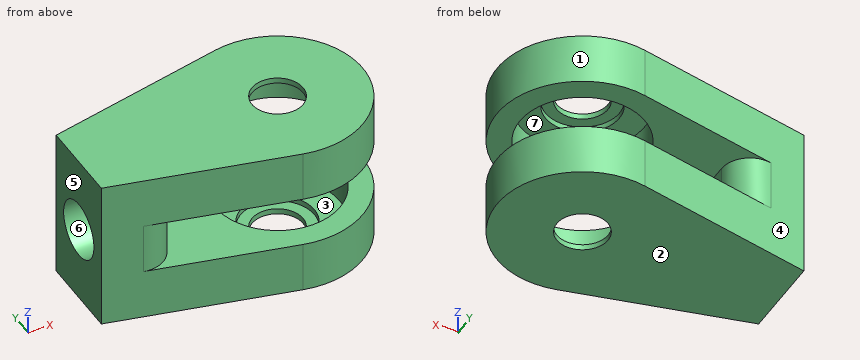
from build123d import *

# Parameters (mm, degrees)
SKETCH1_R               = 15
BOSS_EXTRUDE1_DEPTH     = 9
SKETCH2_R               = 11
CUT_EXTRUDE1_DEPTH      = 7
CUT_EXTRUDE2_REACH      = 40.717
SKETCH3_R               = 4.5
BOSS_EXTRUDE3_REACH     = 44.119
SKETCH6_R               = 5.031250000000002
CUT_EXTRUDE3_DEPTH      = 11.43
FILLET1_R               = 5
CUT_EXTRUDE4_DEPTH      = 1
CUT_EXTRUDE4_DEPTH_BACK = 24
SKETCH7_R               = 6.5


with BuildPart() as part:
    # Sketch1 → Boss-Extrude1 (new body)
    with BuildSketch(Plane.XY):
        with BuildLine():
            ThreePointArc((-3.2926829268292646, -14.634146341463415), (-15, 1.84e-15), (-3.2926829268292708, 14.634146341463413))
            Line((-3.2926829268292703, 14.634146341463419), (-35.00000000000001, 7.499999999999995))
            Line((-35.00000000000001, 7.499999999999995), (-35, -7.500000000000005))
            Line((-35, -7.500000000000005), (-3.292682926829265, -14.634146341463415))
        make_face()
        Circle(SKETCH1_R)
    extrude(amount=BOSS_EXTRUDE1_DEPTH)

    # Sketch2 → Cut-Extrude1 (cut)
    with BuildSketch(Plane.XY.offset(9)):
        Circle(SKETCH2_R)
    extrude(amount=-CUT_EXTRUDE1_DEPTH, mode=Mode.SUBTRACT)

    # Sketch3 → Cut-Extrude2 (cut, up to next)
    with BuildSketch(Plane.XY.offset(2), mode=Mode.PRIVATE) as cut_extrude2_sk1:
        Circle(SKETCH3_R)
    cut_extrude2_tool1 = extrude(cut_extrude2_sk1.sketch, amount=-CUT_EXTRUDE2_REACH, mode=Mode.PRIVATE) & part.part
    add(cut_extrude2_tool1.solids().sort_by_distance((0, 0, 2))[0], mode=Mode.SUBTRACT)


with BuildPart() as body_2:
    # Mirror8: mirrored copy
    add(part.part.mirror(Plane.XY.offset(13.499999999999998)))

    # Sketch4 → Boss-Extrude3 (add, up to next)
    with BuildSketch(Plane.XY.offset(9), mode=Mode.PRIVATE) as boss_extrude3_sk1:
        Polygon((-35.00000000000001, 7.499999999999995), (-35.00000000000001, -7.500000000000005), (-22.300000000000008, -10.357500000000002), (-22.300000000000015, 10.357499999999998), align=None)
    boss_extrude3_tool1 = extrude(boss_extrude3_sk1.sketch, amount=BOSS_EXTRUDE3_REACH, mode=Mode.PRIVATE) - body_2.part

    add(part.part)  # Boss-Extrude3 merges part
    add(boss_extrude3_tool1.solids().sort_by_distance((-28.311298, 0, 9))[0])

    # Sketch6 → Cut-Extrude3 (cut)
    with BuildSketch(Plane.ZY.offset(35.00000000000001)):
        with Locations((13.499999999999998, -3.47e-15)):
            Circle(SKETCH6_R)
    extrude(amount=-CUT_EXTRUDE3_DEPTH, mode=Mode.SUBTRACT)

    # Fillet1
    fillet1_edges = [body_2.edges().sort_by_distance(p)[0] for p in [
        (-22.300000000000015, 10.357499999999996, 13.499999999999998),
        (-22.300000000000008, -10.3575, 13.499999999999998),
    ]]
    fillet(fillet1_edges, radius=FILLET1_R)

    # Sketch7 → Cut-Extrude4 (cut, two sides: drawn at the far end of the back side and taken through both)
    with BuildSketch(Plane.XY.offset(24.999999999999993).offset(-CUT_EXTRUDE4_DEPTH_BACK)):
        Circle(SKETCH7_R)
    extrude(amount=CUT_EXTRUDE4_DEPTH + CUT_EXTRUDE4_DEPTH_BACK, mode=Mode.SUBTRACT)


solid = body_2.part
Design review of the part built by this model. Coordinates are the model's own, in mm. Face numbers are marked on the shaded views. A direction names the side the tool comes from. Round coordinates to 2 decimals unless told otherwise and drop trailing zeros. Order: outer loops, then holes, each group sorted by start corner. A loop starts at its lowest first (then second) coordinate and runs counter-clockwise, first axis right, second up. Notation, with made-up numbers: M -26,72.5 L -5,72.5 A19 ccw -5,80.5 Z; hole C 45,23 d4. An arc over 180 degrees is marked long. Answer as CSV lines item,"result". Start each with the question number.
1) Add section A-A (x = 0). Give the number of separate pieces and of enclosed holes in the cut face, then the cut area to 3 significant figures.
2) Add section C-C (z = 20.75). Give the boundary of the cut face in (x, y), then the cut area to 3 significant figures.
3) Add section B-B (y = 12). Give the boundary of the cut face in (x, z).
4) Wall thickness on line 1 along Z through (x, y) = (-4, -3.5); line 2 along X through (y, z) = (0, 26.65); line 3 along Z through (x, y) = (-21.5, -10.5): over which ranges is each line inside the solid? List them lowest first. Write a range as [from, to].
5) For pin 1 Ø8 at (y, z) = (-2.5, 18.5) entering from +X; pin 2 Ø5 at (y, z) = (-10.5, 8.5) entering from +X; pin 3 Ø6 at (y, z) = (0, 13.5) entering from -X; pin 4 Ø6 at (y, z) = (8.5, 18.5) entering from +X, all flat-tipped, find the tip position at first contact; note any pin that passes through.
6) The part is to be moulded in two halves that separate along Y. For the marked faces 1, 2, 3 and 4, say which applies: +Y half, -Y half, draft (parallel to the pull), parting line (faces both ways), or undercut.
7) Tool access review of the marked faces 5, 6 and 7: name each direction out of +Z, -Z, +X, -X, +Y, -Y from which nothing blocks a thin tool from reaching the whole face with its end or side.
8) Add section D-D (x = -12). Give the boundary of the cut face in (y, z) (3 decimals), then the cut area to 3 significant figures.
Resolved:
1,separate pieces,"4"
1,enclosed holes,"0"
1,area,"188 mm^2"
2,outline,"M -35,-7.5 L -3.29,-14.63 A15 ccw long -3.29,14.63 L -35,7.5 Z; hole C 0,0 d22"
2,area,"773 mm^2"
3,outline,"M -15,0 L 9,0 L 9,9 L -15,9 Z; M -15,18 L 9,18 L 9,27 L -15,27 Z"
4,line 1,"[0, 1], [26, 27]"
4,line 2,"[-35, -4.5], [4.5, 15]"
4,line 3,"[0, 9], [18, 27]"
5,pin 1,"x = 15"
5,pin 2,"x = 12.69"
5,pin 3,"x = -23.57"
5,pin 4,"x = 13.96"
6,face 1,"parting line"
6,face 2,"draft"
6,face 3,"undercut"
6,face 4,"+Y half"
7,face 5,"+Z, -Z, -X, +Y, -Y"
7,face 6,"-X"
7,face 7,"none"
8,outline,"M -12.675,0 L 12.675,0 L 12.675,9 L -12.675,9 Z; M -12.675,18 L 12.675,18 L 12.675,27 L -12.675,27 Z"
8,area,"456 mm^2"
